Could you check a few things on this model? Use its own coordinates, in mm. Face numbers are marked on the shaded views. A direction names the side the tool comes from. Give positions to 0.01 mm unless a question says otherwise; leave off trailing zeros. Loops run counter-clockwise (first coordinate to the right, second up) from the corner with the lowest first, then second, coordinate; pieces in that order, holes last. Notation, with made-up numbers: M 22,10.25 L 73,10.25 A25 ccw 73,47.25 Z; hole C 46,84.5 d3. An arc over 180 degrees is marked long. Answer in a Markdown table with one row per item. Add a question column.
1. I need wall thicknesses on line 1 along X through (y, z) = (0.5, 1.25); line 2 along X through (y, z) = (-1.75, -2.75); line 3 along Z through (x, y) = (-2, -0.75). Which ranges of each line are inside material? Lowest first, please. Write a range as from..to.
2. Thinking about a two-plate mould opening in Z: for the marked faces 4, 5 and 6, which applies, released by +Z, released by -Z, zero draft, split by the parting line, or undercut?
3. If we section it at D-D on x = 1.5: List the corners of the cut face in (y, z) for me, then the cut area to 3 significant figures.
4. I'm going to push flat-ended pins straight in: pin 1 Ø6 at (x, z) = (7.5, -3.5) entering from +Y; pin 2 Ø2.5 at (x, y) = (-2, 0) entering from -Z; pin 3 Ø0.7 at (x, y) = (-2, -0.5) entering from +Z; pin 4 Ø1.5 at (x, y) = (5.5, 4) entering from -Z. Where does each tip first touch, or does it pass through?
5. If we section it at B-B on x = -2: List the corners of the cut face in (y, z) for me.
6. Which directions (+Z, -Z, +X, -X, +Y, -Y) give clear straight access to the entire face, cutting with the end or side of a thin tool? Please do the marked faces 1, 2 and 3.
7. If we section it at A-A on y = 0: List the corners of the cut face in (x, z) for me, then the cut area to 3 significant figures.
8. If we section it at C-C on z = -3.25: List the corners of the cut face in (x, y) for me.
```python
from build123d import *

# Parameters (mm, degrees)
CUT_EXTRUDE_1_DEPTH = 3
FILLET_1_R          = 0.25
CHAMFER_1_SIZE      = 0.5


with BuildPart() as part:
    # Эскиз1 → Повернуть1 (revolve)
    with BuildSketch(Plane.XY):
        with BuildLine():
            Line((0, 5.25), (0, 3))
            Line((0, 3), (10, 3))
            Line((10, 3), (10, 0))
            Line((10, 0), (-3.3, 0))
            Line((-3.3, 0), (-3.3, 4.083197277))
            ThreePointArc((-3.3, 4.083197277), (-1.75010204, 4.949711391), (0, 5.25))
        make_face()
    revolve(axis=Axis((-165.749374514, 0, 0), (1, 0, 0)))

    # Эскиз2 → Вырез-Вытянуть1 (cut)
    with BuildSketch(Plane.ZY.offset(3.3)):
        Polygon((0, -2.309401077), (2, -1.154700538), (2, 1.154700538), (0, 2.309401077), (-2, 1.154700538), (-2, -1.154700538), align=None)
    extrude(amount=-CUT_EXTRUDE_1_DEPTH, mode=Mode.SUBTRACT)

    # Скругление1
    fillet_1_edges = [part.edges().sort_by_distance(p)[0] for p in [
        (-3.3, -1.732050808, -1),
        (-3.3, -1.732050808, 1),
        (-3.3, 0, 2),
        (-3.3, 1.732050808, 1),
        (-3.3, 1.732050808, -1),
        (-3.3, 0, -2),
    ]]
    fillet(fillet_1_edges, radius=FILLET_1_R)

    # Фаска1
    chamfer_1_edges = [part.edges().sort_by_distance(p)[0] for p in [
        (10, -3, 0),
    ]]
    chamfer(chamfer_1_edges, length=CHAMFER_1_SIZE)


solid = part.part
```
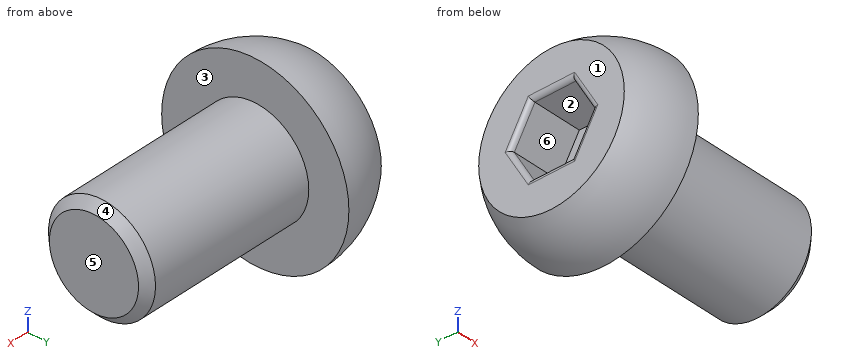
Results:
| question | item | result |
|---|---|---|
| 1 | line 1 | -0.3..10 |
| 1 | line 2 | -3.3..0 |
| 1 | line 3 | -4.8..-2, 2..4.8 |
| 2 | face 4 | split by the parting line |
| 2 | face 5 | zero draft |
| 2 | face 6 | undercut |
| 3 | outline | C 0,0 d6 |
| 3 | area | 28.3 mm2 |
| 4 | pin 1 | y = 2.96 |
| 4 | pin 2 | z = -5.2 |
| 4 | pin 3 | z = 4.96 |
| 4 | pin 4 | through |
| 5 | outline | C 0,0 d9.71; hole M -2.31,0 L -1.15,-2 L 1.15,-2 L 2.31,0 L 1.15,2 L -1.15,2 Z |
| 6 | face 1 | +Z, -Z, -X, +Y, -Y |
| 6 | face 2 | -X |
| 6 | face 3 | +X |
| 7 | outline | M -3.3,-4.08 A5.25 ccw 0,-5.25 L 0,-3 L 9.5,-3 L 10,-2.5 L 10,2.5 L 9.5,3 L 0,3 L 0,5.25 A5.25 ccw -3.3,4.08 L -3.3,2.25 A0.25 ccw -3.05,2 L -0.3,2 L -0.3,-2 L -3.05,-2 A0.25 ccw -3.3,-2.25 Z |
| 7 | area | 79.9 mm2 |
| 8 | outline | M -3.3,-2.47 A4.12 ccw 0,-4.12 L 0,4.12 A4.12 ccw -3.3,2.47 Z |
